Input: part model. Units: mm. Frame: model coordinates. Give positions to 0.01 mm unless a question says otherwise; leave off trailing zeros. Loops run counter-clockwise (first coordinate to the right, second up) from the corner with the lowest first, then second, coordinate; pieces in that order, holes last. Notation, with made-up numbers: (12, 87.25) - (54, 87.25) arc R21 ccw to (54, 91.25) - close; hole circle Ø5 at (19, 85.5). An arc over 180 degrees is marked (long way). Answer as a JSON object with one key per item and string values. Group by question number.
(1) Section query D-D (z = 2.65). Count the separate pieces of the cut face and the enclosed holes in it, plus the area to 3 significant figures.
(2) Pin query (flat end, axial travel): P1, Ø4.5, axis at x = 12.23, y = -38.5, coming from the -Z side (3 decimals); P2, Ø1.5, axis at y = 55.5, z = 3, coming from the -X side; P3, Ø1.5, axis at x = -98, z = 0.5, coming from the -Y side. Return the tip coordinate at first contact, or that it passes through.
(3) Section query B-B (y = -4.5). Return loops of the section in (x, z) (3 decimals).
(4) Mould query, pull axis X, two halves, no side actions, for faces 1 (the cylindrical face through (-52.147, -15.958, 1.565)), 2 (the flat face through (45.288, -95.096, 1.565)), 3 (the flat face through (16, 25, 3.175)), 4 (the flat face through (-64.71, -95.43, 1.57)). Classes: +X half, -X half, draft (parallel to the pull), parting line (faces both ways), or undercut.
(5) Material intervals for L1, parallel to Y at x = -34.5, z = 0.8; L2, parallel to X at y = 40, z = 1.05; L3, parallel to Y at x = 38, z = 2.2, sorted ascending.
(6) Section query A-A (y = 38.5). Return loops of the section in (x, z) (3 decimals), plus the area to 3 significant figures.
(7) Section query C-C (x = -115). Return loops of the section in (y, z) (3 decimals).
```python
from build123d import *

# Parameters (mm, degrees)
SKETCH1_R           = 2.5
SKETCH1_R_2         = 2.6
SKETCH1_R_3         = 1.5
SKETCH1_R_4         = 12.5
SKETCH1_R_5         = 30
BOSS_EXTRUDE1_DEPTH = 3.175
FILLET1_R           = 2
SKETCH3_R           = 1.5
CUT_EXTRUDE1_DEPTH  = 4


with BuildPart() as part:
    # Sketch1 → Boss-Extrude1 (new body)
    with BuildSketch(Plane.XY):
        with BuildLine():
            Line((-120, -25), (-120, 25))
            ThreePointArc((-120, 25), (-94.559451613, 48.820422151), (-86.650635095, 82.762794416))
            Line((-86.650635095, 82.762794416), (-43.349364905, 107.762794416))
            ThreePointArc((-43.349364905, 107.762794416), (-10, 97.640844302), (23.349364905, 107.762794416))
            Line((23.349364905, 107.762794416), (66.650635095, 82.762794416))
            ThreePointArc((66.650635095, 82.762794416), (74.559451613, 48.820422151), (100, 25))
            Line((100, 25), (100, -25))
            ThreePointArc((100, -25), (74.559451613, -48.820422151), (66.650635095, -82.762794416))
            Line((66.650635095, -82.762794416), (23.349364905, -107.762794416))
            ThreePointArc((23.349364905, -107.762794416), (-10, -97.640844302), (-43.349364905, -107.762794416))
            Line((-43.349364905, -107.762794416), (-86.650635095, -82.762794416))
            ThreePointArc((-86.650635095, -82.762794416), (-94.559451613, -48.820422151), (-120, -25))
        make_face()
        with Locations((12.227985364, -38.5)):
            Circle(SKETCH1_R, mode=Mode.SUBTRACT)
        with Locations((-54.455970728, 15)):
            Circle(SKETCH1_R, mode=Mode.SUBTRACT)
        with Locations((12.227985364, 38.5)):
            Circle(SKETCH1_R_2, mode=Mode.SUBTRACT)
        with Locations((-32.227985364, 38.5)):
            Circle(SKETCH1_R_2, mode=Mode.SUBTRACT)
        with Locations((-54.455970728, -15)):
            Circle(SKETCH1_R, mode=Mode.SUBTRACT)
        with Locations((-32.227985364, -38.5)):
            Circle(SKETCH1_R, mode=Mode.SUBTRACT)
        with Locations((95, 15)):
            Circle(SKETCH1_R_2, mode=Mode.SUBTRACT)
        with Locations((95, -15)):
            Circle(SKETCH1_R_2, mode=Mode.SUBTRACT)
        with Locations((-115, -15)):
            Circle(SKETCH1_R_2, mode=Mode.SUBTRACT)
        with Locations((-115, 15)):
            Circle(SKETCH1_R_2, mode=Mode.SUBTRACT)
        with Locations((31.241669751, -97.432667397)):
            Circle(SKETCH1_R, mode=Mode.SUBTRACT)
        with Locations((23.447441117, -101.932667397)):
            Circle(SKETCH1_R, mode=Mode.SUBTRACT)
        with Locations((-43.447441117, -101.932667397)):
            Circle(SKETCH1_R, mode=Mode.SUBTRACT)
        with Locations((-51.241669751, -97.432667397)):
            Circle(SKETCH1_R, mode=Mode.SUBTRACT)
        with Locations((-51.241669751, 97.432667397)):
            Circle(SKETCH1_R, mode=Mode.SUBTRACT)
        with Locations((-43.447441117, 101.932667397)):
            Circle(SKETCH1_R, mode=Mode.SUBTRACT)
        with Locations((23.447441117, 101.932667397)):
            Circle(SKETCH1_R, mode=Mode.SUBTRACT)
        with Locations((31.241669751, 97.432667397)):
            Circle(SKETCH1_R, mode=Mode.SUBTRACT)
        with Locations((34.455970728, -15)):
            Circle(SKETCH1_R, mode=Mode.SUBTRACT)
        with Locations((34.455970728, 15)):
            Circle(SKETCH1_R, mode=Mode.SUBTRACT)
        with Locations((-79, 50)):
            Circle(SKETCH1_R_3, mode=Mode.SUBTRACT)
        with Locations((-60, 50)):
            Circle(SKETCH1_R_3, mode=Mode.SUBTRACT)
        with Locations((-60, -50)):
            Circle(SKETCH1_R_3, mode=Mode.SUBTRACT)
        with Locations((-79, -50)):
            Circle(SKETCH1_R_3, mode=Mode.SUBTRACT)
        with Locations((40, -50)):
            Circle(SKETCH1_R_3, mode=Mode.SUBTRACT)
        with Locations((59, -50)):
            Circle(SKETCH1_R_3, mode=Mode.SUBTRACT)
        with Locations((59, 50)):
            Circle(SKETCH1_R_3, mode=Mode.SUBTRACT)
        with Locations((40, 50)):
            Circle(SKETCH1_R_3, mode=Mode.SUBTRACT)
        with Locations((27.527767497, -65)):
            Circle(SKETCH1_R_4, mode=Mode.SUBTRACT)
        with Locations((-10, 0)):
            Circle(SKETCH1_R_5, mode=Mode.SUBTRACT)
        with Locations((-47.527767497, -65)):
            Circle(SKETCH1_R_4, mode=Mode.SUBTRACT)
        with Locations((-47.527767497, 65)):
            Circle(SKETCH1_R_4, mode=Mode.SUBTRACT)
        with Locations((27.527767497, 65)):
            Circle(SKETCH1_R_4, mode=Mode.SUBTRACT)
        Polygon((-10, 82.640844302), (-13.464101615, 76.640844302), (-6.535898385, 76.640844302), align=None, mode=Mode.SUBTRACT)
    extrude(amount=BOSS_EXTRUDE1_DEPTH)

    # Fillet1
    fillet1_edges = [part.edges().sort_by_distance(p)[0] for p in [
        (-120, -25, 1.5875),
        (-120, 25, 1.5875),
        (-86.650635095, 82.762794416, 1.5875),
        (-43.349364905, 107.762794416, 1.5875),
        (23.349364905, 107.762794416, 1.5875),
        (66.650635095, 82.762794416, 1.5875),
        (100, 25, 1.5875),
        (100, -25, 1.5875),
        (66.650635095, -82.762794416, 1.5875),
        (23.349364905, -107.762794416, 1.5875),
        (-43.349364905, -107.762794416, 1.5875),
        (-86.650635095, -82.762794416, 1.5875),
    ]]
    fillet(fillet1_edges, radius=FILLET1_R)

    # Sketch3 → Cut-Extrude1 (cut)
    with BuildSketch(Plane.XY.offset(3.175)):
        with Locations((-103.5, 16.5)):
            Circle(SKETCH3_R)
        with Locations((-70.5, 16.5)):
            Circle(SKETCH3_R)
        with Locations((-70.5, -16.5)):
            Circle(SKETCH3_R)
        with Locations((-103.5, -16.5)):
            Circle(SKETCH3_R)
        with Locations((50.5, -16.5)):
            Circle(SKETCH3_R)
        with Locations((83.5, -16.5)):
            Circle(SKETCH3_R)
        with Locations((50.5, 16.5)):
            Circle(SKETCH3_R)
        with Locations((83.5, 16.5)):
            Circle(SKETCH3_R)
    extrude(amount=-CUT_EXTRUDE1_DEPTH, mode=Mode.SUBTRACT)


solid = part.part
```
Recorded:
{
 "1": {"separate pieces": "1", "enclosed holes": "42", "area": "30,000 mm^2"},
 "2": {"P1": "passes through", "P2": "stops at x = -91.56", "P3": "stops at y = -44.58"},
 "3": {"outline": "(-120, 0) - (-39.661, 0) - (-39.661, 3.175) - (-120, 3.175) - close; (19.661, 0) - (100, 0) - (100, 3.175) - (19.661, 3.175) - close"},
 "4": {"face 1": "undercut", "face 2": "+X half", "face 3": "draft", "face 4": "-X half"},
 "5": {"L1": "y = -102.87 to -39.54, -37.46 to -17.31, 17.31 to 37.24, 39.76 to 102.87", "L2": "x = -100.77 to -34.35, -30.1 to 10.1, 14.35 to 80.77", "L3": "y = -99.3 to -71.83, -58.17 to 58.17, 71.83 to 99.3"},
 "6": {"outline": "(-102.088, 0) - (-34.828, 0) - (-34.828, 3.175) - (-102.088, 3.175) - close; (-29.628, 0) - (9.628, 0) - (9.628, 3.175) - (-29.628, 3.175) - close; (14.828, 0) - (82.088, 0) - (82.088, 3.175) - (14.828, 3.175) - close", "area": "552 mm^2"},
 "7": {"outline": "(-27.767, 0) - (-17.6, 0) - (-17.6, 3.175) - (-27.767, 3.175) - close; (-12.4, 0) - (12.4, 0) - (12.4, 3.175) - (-12.4, 3.175) - close; (17.6, 0) - (27.767, 0) - (27.767, 3.175) - (17.6, 3.175) - close"}
}
